```python
from build123d import *

# Parameters (mm, degrees)
SKETCH1_W                  = 188
SKETCH1_H                  = 48
BOSS_EXTRUDE1_DEPTH        = 4
SKETCH2_R                  = 1.25
CUT_EXTRUDE1_DEPTH         = 4
CUT_EXTRUDE2_START         = -1.5
SKETCH3_R                  = 2.65
CUT_EXTRUDE2_DEPTH         = 10
M2_TAPPED_HOLE1_AT_2_COUNT = 2
M2_TAPPED_HOLE1_AT_2_PITCH = 9
M2_TAPPED_HOLE1_AT_3_COUNT = 2
M2_TAPPED_HOLE1_AT_3_PITCH = 148
M2_TAPPED_HOLE1_AT_4_COUNT = 2
M2_TAPPED_HOLE1_AT_4_PITCH = 157
CUT_EXTRUDE4_DEPTH         = 98.097888752
CUT_EXTRUDE4_DEPTH_BACK    = 4
SKETCH8_W                  = 19
SKETCH8_H                  = 32
SKETCH9_W                  = 80
SKETCH9_H                  = 32
CUT_EXTRUDE5_DEPTH         = 4
M4_TAPPED_HOLE1_D          = 3.3


with BuildPart() as part:
    # Sketch1 → Boss-Extrude1 (new body)
    with BuildSketch(Plane.XY):
        Rectangle(SKETCH1_W, SKETCH1_H)
    extrude(amount=BOSS_EXTRUDE1_DEPTH)

    # Sketch2 → Cut-Extrude1 (cut)
    with BuildSketch(Plane(origin=(0, 0, 0), x_dir=(-1, 0, 0), z_dir=(0, 0, -1))):
        with Locations((76.5, -20.4)):
            Circle(SKETCH2_R)
        with Locations((82.5, -20.4)):
            Circle(SKETCH2_R)
    cut_extrude1 = extrude(amount=-CUT_EXTRUDE1_DEPTH, mode=Mode.SUBTRACT)

    # Sketch3 → Cut-Extrude2 (cut)
    with BuildSketch(Plane(origin=(0, 0, 0), x_dir=(-1, 0, 0), z_dir=(0, 0, -1)).offset(CUT_EXTRUDE2_START)):
        with Locations((76.5, -20.4)):
            Circle(SKETCH3_R)
        with Locations((82.5, -20.4)):
            Circle(SKETCH3_R)
    cut_extrude2 = extrude(amount=-CUT_EXTRUDE2_DEPTH, mode=Mode.SUBTRACT)

    # Mirror1: Cut-Extrude1, Cut-Extrude2 across plane
    add(cut_extrude1.mirror(Plane(origin=(0, 0, 0), x_dir=(0, 0, 1), z_dir=(0, -1, 0))), mode=Mode.SUBTRACT)
    add(cut_extrude2.mirror(Plane(origin=(0, 0, 0), x_dir=(0, 0, 1), z_dir=(0, -1, 0))), mode=Mode.SUBTRACT)

    # Sketch7 → M2 Tapped Hole1 (revolve, cut)
    with BuildSketch(Plane(origin=(-66, 24, 2), x_dir=(0, 0, 1), z_dir=(1, 0, 0))):
        Polygon((0, 0), (0, 6.480688495), (0.8, 6), (0.8, 0), align=None)
    m2_tapped_hole1 = revolve(axis=Axis((-66, 30.35, 2), (0, -1, 0)), mode=Mode.SUBTRACT)

    # M2 Tapped Hole1 at 2: M2 Tapped Hole1 ×2
    with Locations(*[(i * M2_TAPPED_HOLE1_AT_2_PITCH, 0, 0) for i in range(1, M2_TAPPED_HOLE1_AT_2_COUNT)]):
        add(m2_tapped_hole1, mode=Mode.SUBTRACT)

    # M2 Tapped Hole1 at 3: M2 Tapped Hole1 ×2
    with Locations(*[(i * M2_TAPPED_HOLE1_AT_3_PITCH, 0, 0) for i in range(1, M2_TAPPED_HOLE1_AT_3_COUNT)]):
        add(m2_tapped_hole1, mode=Mode.SUBTRACT)

    # M2 Tapped Hole1 at 4: M2 Tapped Hole1 ×2
    with Locations(*[(i * M2_TAPPED_HOLE1_AT_4_PITCH, 0, 0) for i in range(1, M2_TAPPED_HOLE1_AT_4_COUNT)]):
        add(m2_tapped_hole1, mode=Mode.SUBTRACT)

    # Mirror3: M2 Tapped Hole1 across plane
    add(m2_tapped_hole1.mirror(Plane.ZX), mode=Mode.SUBTRACT)

    # Mirror3 copy 1 sketch → Mirror3 copy 1 (revolve, cut)
    with BuildSketch(Plane(origin=(-57, -24, 2), x_dir=(0, 0, 1), z_dir=(1, 0, 0))):
        Polygon((0, 0), (0, -6.480688495), (0.8, -6), (0.8, 0), align=None)
    revolve(axis=Axis((-57, -30.35, 2), (0, -1, 0)), mode=Mode.SUBTRACT)

    # Mirror3 copy 2 sketch → Mirror3 copy 2 (revolve, cut)
    with BuildSketch(Plane(origin=(82, -24, 2), x_dir=(0, 0, 1), z_dir=(1, 0, 0))):
        Polygon((0, 0), (0, -6.480688495), (0.8, -6), (0.8, 0), align=None)
    revolve(axis=Axis((82, -30.35, 2), (0, -1, 0)), mode=Mode.SUBTRACT)

    # Mirror3 copy 3 sketch → Mirror3 copy 3 (revolve, cut)
    with BuildSketch(Plane(origin=(91, -24, 2), x_dir=(0, 0, 1), z_dir=(1, 0, 0))):
        Polygon((0, 0), (0, -6.480688495), (0.8, -6), (0.8, 0), align=None)
    revolve(axis=Axis((91, -30.35, 2), (0, -1, 0)), mode=Mode.SUBTRACT)

    # Sketch8 → Cut-Extrude4 (cut, two sides: drawn at the far end of the back side and taken through both)
    with BuildSketch(Plane.XY.offset(4).offset(-CUT_EXTRUDE4_DEPTH_BACK)):
        with Locations((79.5, 0)):
            Rectangle(SKETCH8_W, SKETCH8_H)
    extrude(amount=CUT_EXTRUDE4_DEPTH + CUT_EXTRUDE4_DEPTH_BACK, mode=Mode.SUBTRACT)

    # Sketch9 → Cut-Extrude5 (cut)
    with BuildSketch(Plane.XY.offset(4)):
        with Locations((25, 0)):
            Rectangle(SKETCH9_W, SKETCH9_H)
    extrude(amount=-CUT_EXTRUDE5_DEPTH, mode=Mode.SUBTRACT)

    # M4 Tapped Hole1 (through all)
    with Locations(Plane.XY.offset(4)):
        with Locations((-52.5, 16.5), (-26.5, 16.5), (-26.5, -16.5), (-52.5, -16.5)):
            Hole(M4_TAPPED_HOLE1_D / 2)


solid = part.part
```
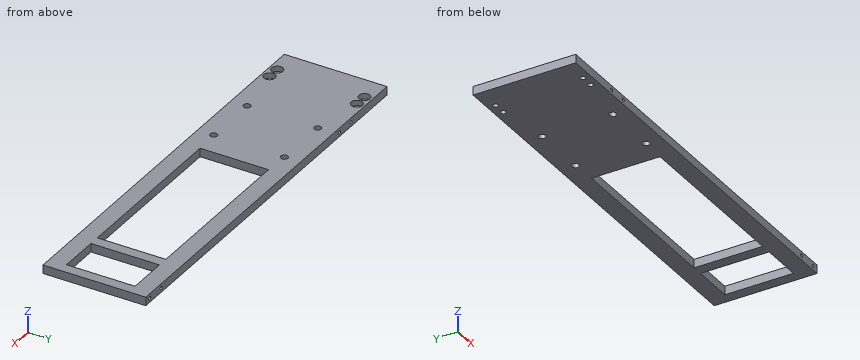
Build history of the part. All positions in model axes, mm. Coordinates: 2 decimals unless noted, no trailing zeros. Order: outer loops, then holes, each group sorted by start corner. A loop starts at its lowest first (then second) coordinate and runs counter-clockwise, first axis right, second up.
Item 1: Saw through at B-B on x = -26.5. List the corners of the cut face in (y, z), then the cut area to 3 significant figures.
Filled in:
outline: (-24, 0) - (-18.15, 0) - (-18.15, 4) - (-24, 4) - close; (-14.85, 0) - (14.85, 0) - (14.85, 4) - (-14.85, 4) - close; (18.15, 0) - (24, 0) - (24, 4) - (18.15, 4) - close
area: 166 mm2
Item 2: Drop flat-ended pins along their axis: pin 1 Ø1.6 at (x, y) = (-77.5, -20) entering from +Z; pin 2 Ø3 at (x, y) = (52, -14) entering from -Z. Give the stop position or say it passes through.
Filled in:
pin 1: stops at z = 1.5
pin 2: passes through
Item 3: Drill centre lines: L1, parallel to X at y = 6.5, z = 3.5; L2, parallel to Y at x = 17, z = 2.95; L3, parallel to Y at x = -76.5, z = 0.7. Where is each one in solid material? Low to high.
Filled in:
L1: x = -94 to -15, 65 to 70, 89 to 94
L2: y = -24 to -16, 16 to 24
L3: y = -24 to -21.65, -19.15 to 19.15, 21.65 to 24
Item 4: Saw through at A-A on y = 7.5. List the corners of the cut face in (x, z).
Filled in:
outline: (-94, 0) - (-15, 0) - (-15, 4) - (-94, 4) - close; (65, 0) - (70, 0) - (70, 4) - (65, 4) - close; (89, 0) - (94, 0) - (94, 4) - (89, 4) - close
